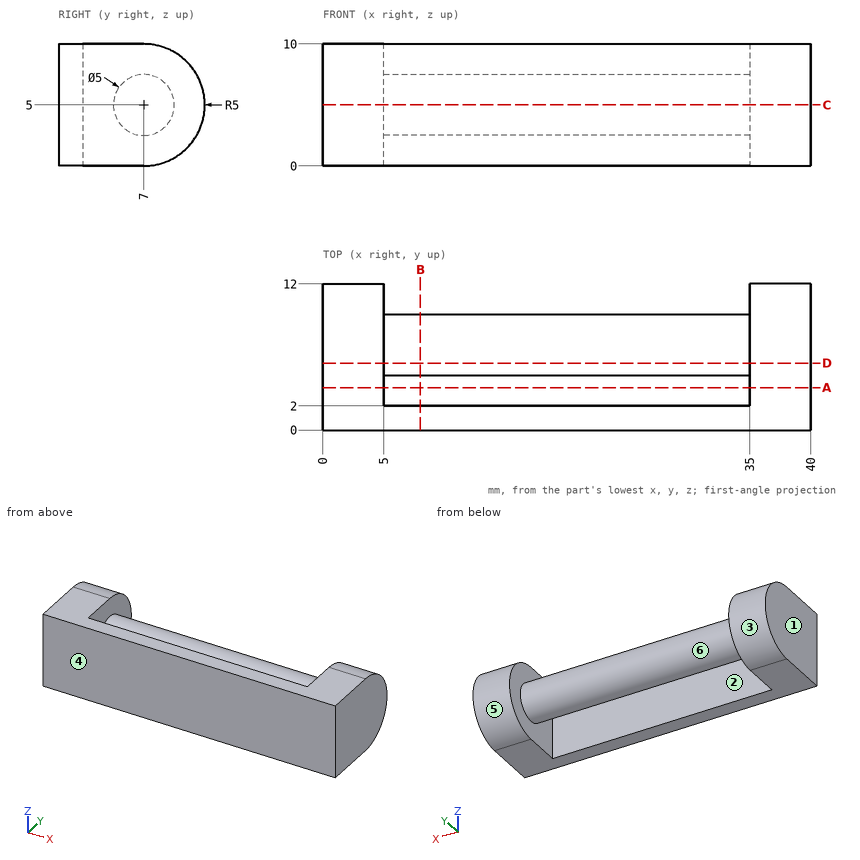
Could you check a few things on this drawing? It's one solid part, dimensions in mm from its lowest x, y, z. A direction names the side the tool comes from. Give positions to 0.01 mm unless a question says otherwise; leave off trailing zeros. Order: outer loops, then holes, each group sorted by start corner. A loop starts at its lowest first (then second) coordinate and runs counter-clockwise, first axis right, second up. Notation, with made-up numbers: (42.5, 88) -> (73.5, 88) arc R10 ccw to (73.5, 100) -> close; hole circle Ø9 at (-11, 22.5). An arc over 180 degrees is marked (long way). Use CSV: the item, a comma, the result in double quotes. Start each with the question number.
Item 1: Suppose I cut it at D-D (y = 5.5). List the corners of the cut face in (x, z) for me, and give its area (3 significant figures).
Item 2: If I drill on probe 1 along X at (y, z) = (2.5, 8.75); probe 2 along Y at (x, z) = (13, 2.75); probe 3 along Y at (x, z) = (28.5, 6.5), over which ranges is the centre line in solid material (lowest first)? Write a range as [from, to].
Item 3: Thinking about a two-plate mould opening in Y: for the marked faces 1, 2, 3 and 4, which applies, pulls with the +Y half, pulls with the -Y half, needs draft (parallel to the pull), parting line crosses it, or undercut?
Item 4: Suppose I cut it at B-B (x = 8). List the corners of the cut face in (y, z) for me.
Item 5: I'm going to push flat-ended pins straight in: P1, Ø2, axis at x = 12.5, z = 2.5, coming from the +Y side; P2, Ø5, axis at x = 10, z = 8.5, coming from the +Y side; P3, Ø4, axis at y = 10.5, z = 5, coming from the -X side; P4, Ø5, axis at x = 25.5, z = 2.5, coming from the +Y side. Where does each tip first touch, or does it pass through?
Item 6: Suppose I cut it at A-A (y = 3.5). List the corners of the cut face in (x, z) for me.
Item 7: Suppose I cut it at C-C (z = 5). List the corners of the cut face in (x, y) for me, and give its area (3 significant figures).
Item 8: On a 3-axis mill with a long thin cutter (end or side, diameter ignored), from which of +Z, -Z, +X, -X, +Y, -Y can I reach the whole of each face in a straight line? I mean the marked faces 5 and 6. Say none if no direction works.
Answer block:
1,outline,"(0, 0) -> (5, 0) -> (5, 3) -> (35, 3) -> (35, 0) -> (40, 0) -> (40, 10) -> (35, 10) -> (35, 7) -> (5, 7) -> (5, 10) -> (0, 10) -> close"
1,area,"220 mm^2"
2,probe 1,"x = [0, 5], [35, 40]"
2,probe 2,"y = [0, 2], [5.91, 8.09]"
2,probe 3,"y = [0, 2], [5, 9]"
3,face 1,"needs draft"
3,face 2,"undercut"
3,face 3,"pulls with the +Y half"
3,face 4,"pulls with the -Y half"
4,outline,"(0, 0) -> (2, 0) -> (2, 10) -> (0, 10) -> close; circle Ø5 at (7, 5)"
5,P1,"stops at y = 9"
5,P2,"stops at y = 9.29"
5,P3,"stops at x = 0"
5,P4,"stops at y = 9.5"
6,outline,"(0, 0) -> (5, 0) -> (5, 10) -> (0, 10) -> close; (35, 0) -> (40, 0) -> (40, 10) -> (35, 10) -> close"
7,outline,"(0, 0) -> (40, 0) -> (40, 12) -> (35, 12) -> (35, 9.5) -> (5, 9.5) -> (5, 12) -> (0, 12) -> close; hole (5, 2) -> (35, 2) -> (35, 4.5) -> (5, 4.5) -> close"
7,area,"330 mm^2"
8,face 5,"+X, -X, +Y"
8,face 6,"none"
